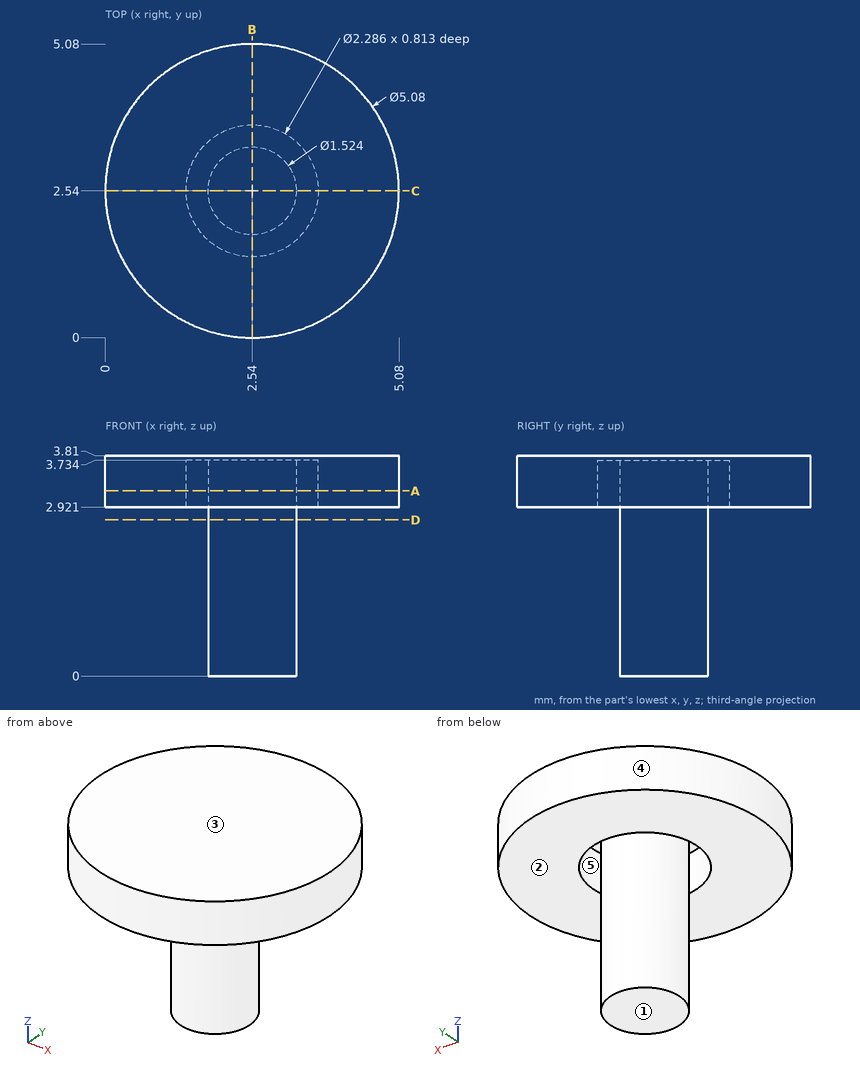
For this review, use the dimensioned drawing (mm, ordinates from the lowest corner) and the shaded views. A direction names the side the tool comes from. Round coordinates to 2 decimals unless told otherwise and drop trailing zeros. Order: outer loops, then holes, each group sorted by start corner. A loop starts at its lowest first (then second) coordinate and runs counter-clockwise, first axis right, second up. Notation, with made-up numbers: M -27,14 L 0,14 A30 cw 0,39 Z; hole C 42.25,22.25 d1. An arc over 180 degrees is marked long. Write each question's results on one line, items separated by ' | '. Start each with the question number.
1. Draft analysis for pull direction X (two halves, no side actions). For the marked faces 3, 4 and 5, state which applies: pulls with the +X half, pulls with the -X half, needs draft (parallel to the pull), parting line crosses it, or undercut.
2. Add section D-D (z = 2.7). State the section outline as (x, y) points.
3. Add section A-A (z = 3.2). State the section outline as (x, y) points.
4. Add section B-B (x = 2.54). State the section outline as (y, z) points.
5. To check wall thickness, follow L1, parallel to Y at x = 2.54, z = 3.4; L2, parallel to Z at x = 4.6, y = 1.9; L3, parallel to X at y = 2.5, z = 2.25. State the ranges of each line that lie inside material, in increasing order. Write a range as [from, to].
6. Tool access review of the marked faces 1 and 2: name each direction out of +Z, -Z, +X, -X, +Y, -Y from which nothing blocks a thin tool from reaching the whole face with its end or side.
7. Clearance check with flat-ended pins moving along their axes: pin 1 Ø1.1 at (x, y) = (3, 2) entering from -Z; pin 2 Ø1 at (y, z) = (1, 3) entering from +X. State where each tip first meets the part, or that it passes through.
Output values:
1) face 3: needs draft | face 4: parting line crosses it | face 5: undercut
2) outline: C 2.54,2.54 d1.52
3) outline: C 2.54,2.54 d5.08; C 2.54,2.54 d1.52; hole C 2.54,2.54 d2.29
4) outline: M 0,2.92 L 1.4,2.92 L 1.4,3.73 L 1.78,3.73 L 1.78,0 L 3.3,0 L 3.3,3.73 L 3.68,3.73 L 3.68,2.92 L 5.08,2.92 L 5.08,3.81 L 0,3.81 Z
5) L1: [0, 1.4], [1.78, 3.3], [3.68, 5.08] | L2: [2.92, 3.81] | L3: [1.78, 3.3]
6) face 1: -Z, +X, -X, +Y, -Y | face 2: -Z
7) pin 1: z = 0 | pin 2: x = 4.86
